Could you check a few things on this model? Use its own coordinates, in mm. A direction names the side the tool comes from. Coordinates: 2 decimals unless noted, no trailing zeros. Write each loop counter-clockwise with the first axis right and the second up, starting at its lowest first coordinate (ties: lowest second). Pieces come first, ordered by that corner, then holes.
Item 1: If I drill on probe 1 along Z at (x, y) = (-59, 5.75); probe 2 along X at (y, z) = (2.5, -2.5); probe 3 along X at (y, z) = (4.3, -70), over which ranges is the centre line in solid material (lowest first)?
Item 2: Thinking about a two-plate mould opening in Z: for faces 1 (the cylindrical face through (0, 3, -60)), 2 (the cylindrical face through (89.03, 2.96, 52.78)), 3 (the cylindrical face through (60, 3, 0)), 4 (the flat face through (85.5, 3, -11.9)), which applies, +Z half, -Z half, draft (parallel to the pull), parting line (faces both ways), or undercut?
Item 3: Which directions (+Z, -Z, +X, -X, +Y, -Y) give clear straight access to the entire face, cutting with the end or side of a thin tool? Please do faces 5 (the cylindrical face through (82.62, 3.04, -23.88)), 6 (the flat face through (92.614, 3.042, 19.18)), 7 (the cylindrical face through (-35.35, 3.04, -48.48)).
Item 4: For P1, Ø5, axis at x = 66.57, z = -21.63, coming from the +Y side; P2, Ø2, axis at x = -12.5, y = 4, coming from the +Z side, each with a flat end and sliding along its axis, tell me the tip position at first contact or that it passes through.
Item 5: I want a section at B-B on z = 0. Please give me the cut outline in (x, y), then the cut area to 3 significant figures.
Item 6: I want a section at A-A on x = 0. Please give me the cut outline in (y, z).
Item 7: I want a section at D-D on y = 2.5. State how many separate pieces and enclosed holes the cut face has, then the cut area to 3 significant figures.
Item 8: I want a section at C-C on x = 68.5. Please give me the cut outline in (y, z).
from build123d import *

# Parameters (mm, degrees)
SKETCH1_R           = 103.5
SKETCH1_R_2         = 60
BOSS_EXTRUDE1_DEPTH = 6
SKETCH2_R           = 4
CUT_EXTRUDE1_DEPTH  = 147.494027182
CIRPATTERN1_COUNT   = 20
SKETCH3_R           = 7.25
CUT_EXTRUDE2_DEPTH  = 6
SKETCH4_OUTSIDE_W   = 267.56
SKETCH4_OUTSIDE_H   = 267.56
CUT_EXTRUDE3_DEPTH  = 147.494027182
CUT_EXTRUDE4_DEPTH  = 10
BOSS_EXTRUDE2_START = -6
BOSS_EXTRUDE2_DEPTH = 6
FILLET1_R           = 6
SKETCH7_R           = 7.5
CUT_EXTRUDE5_DEPTH  = 10


with BuildPart() as part:
    # Sketch1 → Boss-Extrude1 (new body)
    with BuildSketch(Plane(origin=(0, 0, 0), x_dir=(1, 0, 0), z_dir=(0, 1, 0))):
        with Locations(Location((0, 0, 0), (0, 0, 270))):
            Circle(SKETCH1_R)
        with Locations(Location((0, 0, 0), (0, 0, 270))):
            Circle(SKETCH1_R_2, mode=Mode.SUBTRACT)
    extrude(amount=BOSS_EXTRUDE1_DEPTH)

    # Sketch2 → Cut-Extrude1 (cut, through all)
    with BuildSketch(Plane(origin=(0, 6, 0), x_dir=(1, 0, 0), z_dir=(0, 1, 0))):
        with Locations(Location((0, 70, 0), (0, 0, 270))):
            Circle(SKETCH2_R)
    cut_extrude1 = extrude(amount=-CUT_EXTRUDE1_DEPTH, mode=Mode.SUBTRACT)

    # CirPattern1: Cut-Extrude1 ×20 about axis
    cirpattern1_axis = Axis((0, 0, 0), (0, 1, 0))
    for i in range(1, CIRPATTERN1_COUNT):
        add(cut_extrude1.rotate(cirpattern1_axis, i * 360 / CIRPATTERN1_COUNT), mode=Mode.SUBTRACT)

    # Sketch3 → Cut-Extrude2 (cut)
    with BuildSketch(Plane(origin=(0, 6, 0), x_dir=(1, 0, 0), z_dir=(0, 1, 0))):
        with Locations(Location((86.266964059, -36.13705179, 0), (0, 0, 270))):
            Circle(SKETCH3_R)
        with Locations(Location((73.328010939, -58.059266372, 0), (0, 0, 270))):
            Circle(SKETCH3_R)
    extrude(amount=-CUT_EXTRUDE2_DEPTH, mode=Mode.SUBTRACT)

    # Sketch4 outside → Cut-Extrude3 (cut, through all)
    with BuildSketch(Plane(origin=(0, 6, 0), x_dir=(1, 0, 0), z_dir=(0, 1, 0))):
        Rectangle(SKETCH4_OUTSIDE_W, SKETCH4_OUTSIDE_H)
        with BuildLine():
            Line((23.716937817, -82.665028038), (76.077499384, -67.64256676))
            ThreePointArc((76.077499384, -67.64256676), (78.876917409, -66.342319555), (81.144475094, -64.248145201))
            ThreePointArc((81.144475094, -64.248145201), (89.13274289, -52.60802358), (95.46266736, -39.989112774))
            ThreePointArc((95.46266736, -39.989112774), (96.200172038, -36.991868886), (95.985582928, -33.91269114))
            Line((95.985582928, -33.91269114), (83.832277903, 19.187214014))
            ThreePointArc((83.832277903, 19.187214014), (-74.061989261, 43.712947129), (23.716937817, -82.665028038))
        make_face(mode=Mode.SUBTRACT)
    extrude(amount=-CUT_EXTRUDE3_DEPTH, mode=Mode.SUBTRACT)

    # Sketch5 → Cut-Extrude4 (cut)
    with BuildSketch(Plane(origin=(0, 6, 0), x_dir=(1, 0, 0), z_dir=(0, 1, 0))):
        with BuildLine():
            ThreePointArc((46.694681279, 42.270046437), (48.541019662, 35.267115138), (54.63065317, 31.347118204))
            ThreePointArc((54.63065317, 31.347118204), (57.394464692, 29.243940421), (57.471443608, 25.771753046))
            ThreePointArc((57.471443608, 25.771753046), (57.063390978, 18.541019662), (61.643630936, 12.931080792))
            ThreePointArc((61.643630936, 12.931080792), (63.622254217, 10.076775126), (62.622500611, 6.750740904))
            ThreePointArc((62.622500611, 6.750740904), (60, 0), (62.622500611, -6.750740904))
            ThreePointArc((62.622500611, -6.750740904), (63.622254217, -10.076775126), (61.643630936, -12.931080792))
            ThreePointArc((61.643630936, -12.931080792), (57.063390978, -18.541019662), (57.471443608, -25.771753046))
            ThreePointArc((57.471443608, -25.771753046), (57.394464692, -29.243940421), (54.63065317, -31.347118204))
            ThreePointArc((54.63065317, -31.347118204), (48.541019662, -35.267115138), (46.694681279, -42.270046437))
            ThreePointArc((46.694681279, -42.270046437), (45.548505072, -45.548505072), (42.270046437, -46.694681279))
            ThreePointArc((42.270046437, -46.694681279), (35.267115138, -48.541019662), (31.347118204, -54.63065317))
            ThreePointArc((31.347118204, -54.63065317), (29.243940421, -57.394464692), (25.771753046, -57.471443608))
            ThreePointArc((25.771753046, -57.471443608), (18.541019662, -57.063390978), (12.931080792, -61.643630936))
            ThreePointArc((12.931080792, -61.643630936), (10.076775126, -63.622254217), (6.750740904, -62.622500611))
            ThreePointArc((6.750740904, -62.622500611), (0, -60), (-6.750740904, -62.622500611))
            ThreePointArc((-6.750740904, -62.622500611), (-10.076775126, -63.622254217), (-12.931080792, -61.643630936))
            ThreePointArc((-12.931080792, -61.643630936), (-18.541019662, -57.063390978), (-25.771753046, -57.471443608))
            ThreePointArc((-25.771753046, -57.471443608), (-29.243940421, -57.394464692), (-31.347118204, -54.63065317))
            ThreePointArc((-31.347118204, -54.63065317), (-35.267115138, -48.541019662), (-42.270046437, -46.694681279))
            ThreePointArc((-42.270046437, -46.694681279), (-45.548505072, -45.548505072), (-46.694681279, -42.270046437))
            ThreePointArc((-46.694681279, -42.270046437), (-48.541019662, -35.267115138), (-54.63065317, -31.347118204))
            ThreePointArc((-54.63065317, -31.347118204), (-57.394464692, -29.243940421), (-57.471443608, -25.771753046))
            ThreePointArc((-57.471443608, -25.771753046), (-57.063390978, -18.541019662), (-61.643630936, -12.931080792))
            ThreePointArc((-61.643630936, -12.931080792), (-63.622254217, -10.076775126), (-62.622500611, -6.750740904))
            ThreePointArc((-62.622500611, -6.750740904), (-60, 0), (-62.622500611, 6.750740904))
            ThreePointArc((-62.622500611, 6.750740904), (-63.622254217, 10.076775126), (-61.643630936, 12.931080792))
            ThreePointArc((-61.643630936, 12.931080792), (-57.063390978, 18.541019662), (-57.471443608, 25.771753046))
            ThreePointArc((-57.471443608, 25.771753046), (-57.394464692, 29.243940421), (-54.63065317, 31.347118204))
            ThreePointArc((-54.63065317, 31.347118204), (-48.541019662, 35.267115138), (-46.694681279, 42.270046437))
            ThreePointArc((-46.694681279, 42.270046437), (-45.548505072, 45.548505072), (-42.270046437, 46.694681279))
            ThreePointArc((-42.270046437, 46.694681279), (-35.267115138, 48.541019662), (-31.347118204, 54.63065317))
            ThreePointArc((-31.347118204, 54.63065317), (-29.243940421, 57.394464692), (-25.771753046, 57.471443608))
            ThreePointArc((-25.771753046, 57.471443608), (-18.541019662, 57.063390978), (-12.931080792, 61.643630936))
            ThreePointArc((-12.931080792, 61.643630936), (-10.076775126, 63.622254217), (-6.750740904, 62.622500611))
            ThreePointArc((-6.750740904, 62.622500611), (0, 60), (6.750740904, 62.622500611))
            ThreePointArc((6.750740904, 62.622500611), (10.076775126, 63.622254217), (12.931080792, 61.643630936))
            ThreePointArc((12.931080792, 61.643630936), (18.541019662, 57.063390978), (25.771753046, 57.471443608))
            ThreePointArc((25.771753046, 57.471443608), (29.243940421, 57.394464692), (31.347118204, 54.63065317))
            ThreePointArc((31.347118204, 54.63065317), (35.267115138, 48.541019662), (42.270046437, 46.694681279))
            ThreePointArc((42.270046437, 46.694681279), (45.548505072, 45.548505072), (46.694681279, 42.270046437))
        make_face()
    extrude(amount=-CUT_EXTRUDE4_DEPTH, mode=Mode.SUBTRACT)

    # Sketch6 → Boss-Extrude2 (add)
    with BuildSketch(Plane.XZ.offset(BOSS_EXTRUDE2_START)):
        with BuildLine():
            Line((8.989447841, 85.528883002), (-17.398199941, 88.302336542))
            ThreePointArc((-17.398199941, 88.302336542), (-69.870812829, -56.728031119), (82.845436811, -35.165801564))
            Line((82.845436811, -35.165801564), (79.163417397, -33.60287705))
            ThreePointArc((79.163417397, -33.60287705), (-74.100107798, -43.648299215), (8.989447841, 85.528883002))
        make_face()
    extrude(amount=BOSS_EXTRUDE2_DEPTH)

    # Fillet1
    # the kernel refuses this fillet: 6 mm, written as the material it adds along each edge
    with BuildSketch(Plane(origin=(79.163417397, 6, -33.60287705), x_dir=(0.3619298171455144, 0, 0.9322053461877455), z_dir=(0, -1, 0))) as fillet1_piece_1:
        with BuildLine():
            CenterArc((5.532861862, -5.997100749), FILLET1_R, 91.781239909, 68.757327573)
            Line((-0.124333974, -3.998067166), (-0.237477891, -3.958086494))
            ThreePointArc((-0.237477891, -3.958086494), (-0.182109002, -1.995303564), (-0.119942015, 0.003730019))
            Line((-0.119942015, 0.003730019), (0.003730019, 0.119942015))
            ThreePointArc((0.003730019, 0.119942015), (2.67318045, 0.078444066), (5.342630881, 0.119942015))
            Line((5.342630881, 0.119942015), (5.346360901, 0))
        make_face()
    extrude(amount=6)

    # Sketch7 → Cut-Extrude5 (cut)
    with BuildSketch(Plane.XZ):
        with Locations((94.002430013, -1.686361811)):
            Circle(SKETCH7_R)
    extrude(amount=-CUT_EXTRUDE5_DEPTH, mode=Mode.SUBTRACT)


solid = part.part
Response values:
1. probe 1: z = -67.96 to -44.37, -37.92 to -15.1, 15.1 to 37.92, 44.37 to 67.96
1. probe 2: x = -89.97 to -73.12, -66.88 to -60.32, 60.32 to 66.88, 73.12 to 86.55
1. probe 3: x = -56.57 to -23.7, -19.57 to -4, 4 to 19.57, 23.7 to 56.57
2. face 1: undercut
2. face 2: +Z half
2. face 3: undercut
2. face 4: -Z half
3. face 5: +X, +Y, -Y
3. face 6: -Z, +X, +Y, -Y
3. face 7: +Y, -Y
4. P1: passes through
4. P2: stops at z = 87.89
5. outline: (-90, 0) - (-74, 0) - (-74, 6) - (-90, 6) - close; (-66, 0) - (-60, 0) - (-60, 6) - (-66, 6) - close; (60, 0) - (66, 0) - (66, 6) - (60, 6) - close; (74, 0) - (86.69, 0) - (86.69, 6) - (74, 6) - close
5. area: 244 mm2
6. outline: (0, -90) - (6, -90) - (6, -74) - (0, -74) - close; (0, -66) - (6, -66) - (6, -60) - (0, -60) - close; (0, 60) - (6, 60) - (6, 66) - (0, 66) - close; (0, 74) - (6, 74) - (6, 86.47) - (0, 86.47) - close
7. separate pieces: 1
7. enclosed holes: 23
7. area: 12,500 mm2
8. outline: (0, -58.38) - (6, -58.38) - (6, -25.14) - (0, -25.14) - close; (0, -18.13) - (6, -18.13) - (6, -3.71) - (0, -3.71) - close; (0, 3.71) - (6, 3.71) - (6, 18.13) - (0, 18.13) - close; (0, 25.14) - (6, 25.14) - (6, 52.65) - (0, 52.65) - close; (0, 63.47) - (6, 63.47) - (6, 69.82) - (0, 69.82) - close
